For this review, take the finished solid that the model builds, in its own axes (mm). Face numbers are marked on the shaded views. A direction names the side the tool comes from. Give positions to 0.01 mm unless a question says otherwise; leave off trailing zeros. Write each loop counter-clockwise with the first axis right and the second up, starting at its lowest first coordinate (ties: lowest second). Pieces come first, ordered by that corner, then holes. Notation, with made-up numbers: M 64.5,47.5 L 77.5,47.5 A18 ccw 77.5,59.5 Z; hole C 61.25,32.25 d6. An arc over 180 degrees is marked long. Answer as a JSON object with one key per item and string values. Group by question number.
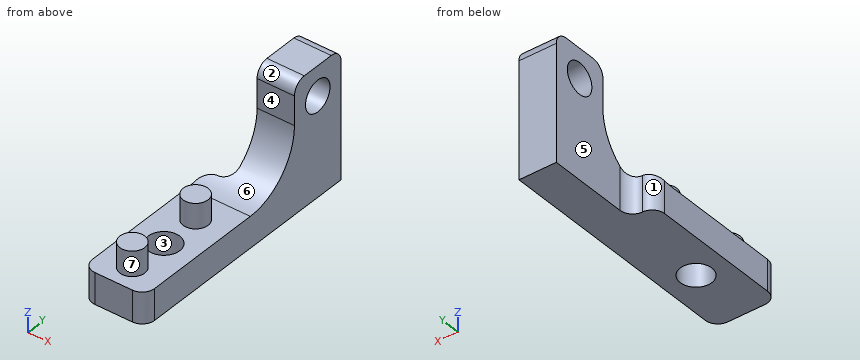
Autodesk Inventor part; units mm, degrees
ref_plane "YZ Plane" through (0, 0, 0) normal (1, 0, 0) x (0, 1, 0)
ref_plane "XZ Plane" through (0, 0, 0) normal (0, 1, 0) x (-1, 0, 0)
ref_plane "XY Plane" through (0, 0, 0) normal (0, 0, 1) x (1, 0, 0)
sketch "Sketch1" plane through (0, 0, 0) normal (1, 0, 0) x (0, 1, 0)
  line L0 (0, 0) -> (15.25, 0)
  line L1 (15.25, 0) -> (15.25, 7.825)
  line L2 (15.25, 7.825) -> (20, 7.825)
  line L3 (20, 7.825) -> (20, -2.5)
  line L4 (20, -2.5) -> (0, -2.5)
  line L5 (0, -2.5) -> (0, 0)
  point P0 (17.625, 5.45)
  dimension "d8" = 2.5
  dimension "d21" = 5.45
  dimension "d23" = 20
  dimension "d24" = 2.375
  dimension "d25" = 2.375
  dimension "d26" = 2.375
extrude "Extrusion1" add sketch "Sketch1" along normal blind 5
sketch "Sketch2" plane through (0, 0, 0) normal (0, 0, 1) x (1, 0, 0)
  line L0 (2.5, 1.9) -> (2.5, 8.35) construction
  line L1 (5, 15.25) -> (5, 0) construction
  line L2 (0, 0) -> (0, 15.25) construction
  circle A0 centre (2.5, 8.35) radius 1
  circle A1 centre (2.5, 1.9) radius 1
  line L3 (0, 0) -> (5, 0)
  line L4 (0, 15.25) -> (5, 15.25)
  point P0 (2.5, 5.125)
  dimension "d2" = 5
  dimension "d3" = 2.5
  dimension "d4" = 8.45
  dimension "d5" = 2
  dimension "d6" = 2
  dimension "d27" = 5.125
extrude "Extrusion2" add sketch "Sketch2" along normal blind 2
hole "Hole1" at (2.5, 5.125, 0) direction (0, 0, -1) diameter 2.53 end through all
fillet "Fillet1" radius 1 2 edges at (5, 0, -1.25) (0, 0, -1.25)
sketch "Sketch3" plane through (5, 20, -2.5) normal (0, 0, -1) x (-1, 0, 0)
  line L0 (5, 0) -> (5, -19)
  line L1 (5, 0) -> (3, 0)
  line L2 (3, 0) -> (3, -7.5)
  line L3 (3, -7.5) -> (5, -7.5)
  line L4 (5, -7.5) -> (5, 0)
  line L5 (0, -19) -> (0, 0)
  point P0 (5, -20)
  dimension "d28" = 3
  dimension "d29" = 7.5
extrude "Extrusion3" cut sketch "Sketch3" against normal up to surface (10.325 mm away)
hole "Hole2" at (0, 17.625, 5.45) direction (1, 0, 0) diameter 2.5 end through all
fillet "Fillet2" radius 1 4 edges at (0, 12.5, -1.25) (2, 12.5, -1.25) (3.5, 15.25, 7.825) (3.5, 20, 7.825)
fillet "Fillet2" radius 4.5 1 edges at (3.5, 15.25, 0)
equation "\"d3\" = 0.5 * d2"
equation "\"d6\" = d5"
properties part number "BR"
Item 1: Draft analysis for pull direction X (two halves, no side actions). For the marked faces 1, 2 and 3, state which applies: released by +X, released by -X, zero draft, split by the parting line, or undercut.
Item 2: Consider section D-D (y = 8.35). Give the boundary of the cut face in (x, z).
Item 3: Consider section C-C (z = 5.45). Give the boundary of the cut face in (x, y) (3 decimals), plus the area to 3 significant figures.
Item 4: To check wall thickness, follow probe 1 along Y at (x, z) = (3.85, 5.45) (3 decimals); probe 2 along Y at (x, z) = (2.5, -0.65); probe 3 along X at (y, z) = (17.25, -1.25). State the ranges of each line that lie inside material, in increasing order.
Item 5: Insertion check: P1, Ø1.2, axis at x = 3, z = 6, coming from the -Y side; P2, Ø3, axis at x = 1.5, z = 0.5, coming from the +Y side; P3, Ø3.5, axis at y = 18, z = 4.5, coming from the -X side; P4, Ø2, axis at x = 2.5, y = 8.5, coming from the +Z side. Each pin has a flat end and moves straight along its axis. Give the tip position at first contact, or say it passes through.
Item 6: Consider section B-B (x = 2.5). Give the boundary of the cut face in (y, z) (3 decimals), plus the area to 3 significant figures.
Item 7: Machinability: for the marked faces 4, 5, 6 and 7, which of the approach directions +Z, -Z, +X, -X, +Y, -Y give a long, thin tool a straight path to every point of the face, cutting with its end or side? Answer none if there is none.
Result set:
{
 "1": {"face 1": "released by -X", "face 2": "zero draft", "face 3": "undercut"},
 "2": {"outline": "M 0,-2.5 L 5,-2.5 L 5,0 L 3.5,0 L 3.5,2 L 1.5,2 L 1.5,0 L 0,0 Z"},
 "3": {"outline": "M 2,15.25 L 5,15.25 L 5,16.375 L 2,16.375 Z; M 2,18.875 L 5,18.875 L 5,20 L 2,20 Z", "area": "6.75 mm^2"},
 "4": {"probe 1": "y = 15.25 to 16.375, 18.875 to 20", "probe 2": "y = 0 to 3.86, 6.39 to 20", "probe 3": "x = 2 to 5"},
 "5": {"P1": "stops at y = 15.25", "P2": "stops at y = 20", "P3": "stops at x = 2", "P4": "stops at z = 2"},
 "6": {"outline": "M 0,-2.5 L 3.86,-2.5 L 3.86,0 L 2.9,0 L 2.9,2 L 0.9,2 L 0.9,0 L 0,0 Z; M 6.39,-2.5 L 20,-2.5 L 20,6.825 A1 ccw 19,7.825 L 16.25,7.825 A1 ccw 15.25,6.825 L 15.25,4.5 A4.5 cw 10.75,0 L 9.35,0 L 9.35,2 L 7.35,2 L 7.35,0 L 6.39,0 Z; hole C 17.625,5.45 d2.5", "area": "87.9 mm^2"},
 "7": {"face 4": "+Z, +X, -X, -Y", "face 5": "+Z, -Z, -X, +Y", "face 6": "+Z, +X, -X", "face 7": "+Z"}
}
